Source: CAD feature listing. Evaluate the final solid. Frame: model axes, mm. Face numbers are marked on the shaded views. A direction names the side the tool comes from. Give positions to 0.01 mm unless a question says otherwise; leave off trailing zeros. Loops run counter-clockwise (first coordinate to the right, second up) from the corner with the lowest first, then second, coordinate; pieces in that order, holes last. Notation, with made-up numbers: (-13, -2.5) -> (17, -2.5) arc R13 cw to (17, 10.5) -> close; hole circle Ø9 at (17, -20.5). An arc over 180 degrees is marked (long way). Return JSON: item names as keys, results as strings. Group by question number.
(1) Access query for the marked faces 5 and 6. Directions: +Z, -Z, +X, -X, +Y, -Y. A direction counts if a zero-diameter tool reaches every point of the face in a straight line with its end or side. Return the directions, or none.
(2) Draft query along Y for the marked faces 1, 2, 3 and 4. Return one class per face: released by +Y, released by -Y, zero draft, split by the parting line, or undercut.
(3) Cut plane B-B on x = 4.5. Return loops of the section in (y, z), then the cut area to 3 significant figures.
(4) Pin query (flat end, axial travel): pin 1 (12 mm diameter, centred on x = -12, y = -10, fed in from +Z). Return the tip coordinate at first contact, or that it passes through.
(5) Cut plane C-C on y = 16. Return loops of the section in (x, z).
(6) Cut plane A-A on z = 17.5. Return loops of the section in (x, y), then the cut area to 3 significant figures.
(7) Ray query, line 1 (Y direction, x = -8.5, z = 3.5); line 2 (X direction, y = 23, z = 22); line 3 (Z direction, x = -16, y = -3). Return the intervals inside material, ascending. Write a range as from..to.
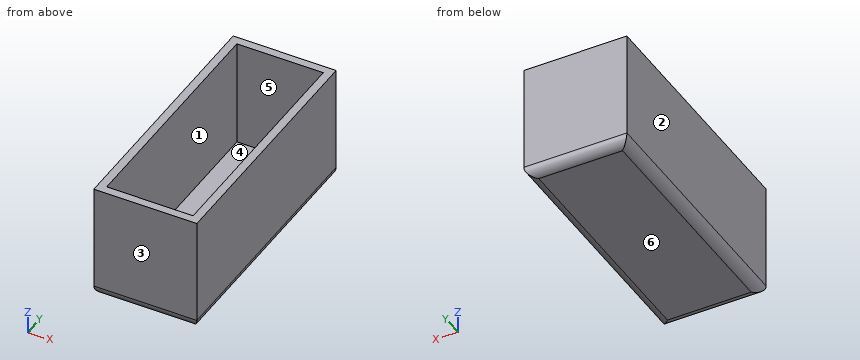
```python
from build123d import *

# Parameters (mm, degrees)
F0_W     = 31
F0_H     = 76
F1_DEPTH = 35
F2_T     = -2.5
F3_R     = 2.9


with BuildPart() as f1:
    # F0 (on Top) → F1 (new body)
    with BuildSketch(Plane.XY):
        with Locations((-5.62528, -5.040663)):
            Rectangle(F0_W, F0_H)
    extrude(amount=F1_DEPTH)

    # F2
    f2_openings = [f1.faces().sort_by_distance(p)[0] for p in [
        (-5.62528, -5.040663, 35),
    ]]
    offset(amount=F2_T, openings=f2_openings)

    # F3
    f3_edges = [f1.edges().sort_by_distance(p)[0] for p in [
        (-5.62528, -43.040663, 0),
        (9.87472, -5.040663, 0),
        (-21.12528, -5.040663, 0),
        (-5.62528, 32.959337, 0),
    ]]
    fillet(f3_edges, radius=F3_R)


solid = f1.part
```
Answers:
{
 "1": {"face 5": "+Z", "face 6": "-Z, +X, -X, +Y, -Y"},
 "2": {"face 1": "undercut", "face 2": "zero draft", "face 3": "released by -Y", "face 4": "undercut"},
 "3": {"outline": "(-43.04, 2.9) arc R2.9 ccw to (-40.14, 0) -> (30.06, 0) arc R2.9 ccw to (32.96, 2.9) -> (32.96, 35) -> (30.46, 35) -> (30.46, 2.5) -> (-40.54, 2.5) -> (-40.54, 35) -> (-43.04, 35) -> close", "area": "349 mm²"},
 "4": {"pin 1": "z = 2.5"},
 "5": {"outline": "(-21.13, 2.9) arc R2.9 ccw to (-18.23, 0) -> (6.97, 0) arc R2.9 ccw to (9.87, 2.9) -> (9.87, 35) -> (7.37, 35) -> (7.37, 2.5) -> (-18.63, 2.5) -> (-18.63, 35) -> (-21.13, 35) -> close"},
 "6": {"outline": "(-21.13, -43.04) -> (9.87, -43.04) -> (9.87, 32.96) -> (-21.13, 32.96) -> close; hole (-18.63, -40.54) -> (7.37, -40.54) -> (7.37, 30.46) -> (-18.63, 30.46) -> close", "area": "510 mm²"},
 "7": {"line 1": "-43.04..-40.54, 30.46..32.96", "line 2": "-21.13..-18.63, 7.37..9.87", "line 3": "0..2.5"}
}
